Autodesk Inventor part; units mm, degrees
ref_plane "YZ Plane" through (0, 0, 0) normal (1, 0, 0) x (0, 1, 0)
ref_plane "XZ Plane" through (0, 0, 0) normal (0, 1, 0) x (-1, 0, 0)
ref_plane "XY Plane" through (0, 0, 0) normal (0, 0, 1) x (1, 0, 0)
sketch "スケッチ1" plane through (0, 0, 0) normal (0, 0, 1) x (1, 0, 0)
  circle A0 centre (0, 0) radius 1.6
  circle A1 centre (10, 0) radius 1.6
  circle A2 centre (-10, 0) radius 1.6
  circle A3 centre (0, 18) radius 1.6
  circle A4 centre (0, 38) radius 1.6
  circle A5 centre (0, 28) radius 1.6
  line L0 (-17.5, 7.5) -> (-17.5, -7.5)
  line L1 (-17.5, -7.5) -> (17.5, -7.5)
  line L2 (17.5, -7.5) -> (17.5, 7.5)
  line L3 (17.5, 7.5) -> (7.5, 45.5)
  line L4 (7.5, 45.5) -> (-7.5, 45.5)
  line L5 (-7.5, 45.5) -> (-17.5, 7.5)
  dimension "d0" = 3.2
  dimension "d1" = 3.2
  dimension "d2" = 3.2
  dimension "d3" = 10
  dimension "d4" = 10
  dimension "d5" = 3.2
  dimension "d6" = 3.2
  dimension "d7" = 3.2
  dimension "d8" = 18
  dimension "d9" = 10
  dimension "d10" = 10
  dimension "d11" = 7.5
  dimension "d12" = 7.5
  dimension "d13" = 7.5
  dimension "d14" = 7.5
  dimension "d15" = 7.5
  dimension "d16" = 7.5
  dimension "d17" = 7.5
extrude "押し出し1" add sketch "スケッチ1" along normal blind 3
fillet "フィレット1" radius 2 6 edges at (-7.5, 45.5, 1.5) (7.5, 45.5, 1.5) (17.5, 7.5, 1.5) (17.5, -7.5, 1.5) (-17.5, -7.5, 1.5) (-17.5, 7.5, 1.5)
properties part number "オムニ_固定具5" material "アルミニウム 6061"
Geometry check sheet. Reference: the model listing, model coordinates, mm. Round coordinates to 2 decimals unless told otherwise and drop trailing zeros. Loops run counter-clockwise (first coordinate to the right, second up) from the corner with the lowest first, then second, coordinate; pieces in that order, holes last. Notation, with made-up numbers: (-19, 72.5) -> (19, 72.5) arc R33 ccw to (19, 104.5) -> close; hole circle Ø9 at (55, -16.75). An arc over 180 degrees is marked (long way). Use a Markdown table: item, result.
(1) Mould release check, pull along X, two halves, no side actions. Record for faces 1 (the flat face through (12.73, 25.63, 1.48)), 2 (the flat face through (-17.5, 1, 1)), 3 (the cylindrical face through (-11.6, -0.07, 1.48)): released by +X, released by -X, zero draft, split by the parting line, or undercut.
Calculated:
| item | result |
|---|---|
| face 1 | released by +X |
| face 2 | released by -X |
| face 3 | undercut |
(2) Sectioned sample at D-D (y = 33.5). Enter the section's corners in (x, z).
Calculated:
| item | result |
|---|---|
| outline | (-10.66, 0) -> (10.66, 0) -> (10.66, 3) -> (-10.66, 3) -> close |
(3) Sectioned sample at C-C (x = 10). Enter the section's corners in (y, z).
Calculated:
| item | result |
|---|---|
| outline | (-7.5, 0) -> (-1.6, 0) -> (-1.6, 3) -> (-7.5, 3) -> close; (1.6, 0) -> (36, 0) -> (36, 3) -> (1.6, 3) -> close |
(4) Sectioned sample at B-B (z = 1.45). Enter the section's corners in (x, y), then the cut area to 3 significant figures.
Calculated:
| item | result |
|---|---|
| outline | (-17.5, -5.5) arc R2 ccw to (-15.5, -7.5) -> (15.5, -7.5) arc R2 ccw to (17.5, -5.5) -> (17.5, 7.24) arc R2 ccw to (17.43, 7.75) -> (7.89, 44.01) arc R2 ccw to (5.96, 45.5) -> (-5.96, 45.5) arc R2 ccw to (-7.89, 44.01) -> (-17.43, 7.75) arc R2 ccw to (-17.5, 7.24) -> close; hole circle Ø3.2 at (-10, 0); hole circle Ø3.2 at (0, 0); hole circle Ø3.2 at (0, 18); hole circle Ø3.2 at (0, 28); hole circle Ø3.2 at (0, 38); hole circle Ø3.2 at (10, 0) |
| area | 1,420 mm² |
(5) Scan lines: probe 1 along Y at (x, z) = (0, 1.95); probe 2 along X at (y, z) = (39, 2.4); probe 3 along X at (y, z) = (12, 1.95). Record each from-to range of solid material in increasing order.
Calculated:
| item | result |
|---|---|
| probe 1 | -7.5 to -1.6, 1.6 to 16.4, 19.6 to 26.4, 29.6 to 36.4, 39.6 to 45.5 |
| probe 2 | -9.21 to -1.25, 1.25 to 9.21 |
| probe 3 | -16.32 to 16.32 |
(6) Sectioned sample at A-A (x = 0). Enter the section's corners in (y, z), then the cut area to 3 significant figures.
Calculated:
| item | result |
|---|---|
| outline | (-7.5, 0) -> (-1.6, 0) -> (-1.6, 3) -> (-7.5, 3) -> close; (1.6, 0) -> (16.4, 0) -> (16.4, 3) -> (1.6, 3) -> close; (19.6, 0) -> (26.4, 0) -> (26.4, 3) -> (19.6, 3) -> close; (29.6, 0) -> (36.4, 0) -> (36.4, 3) -> (29.6, 3) -> close; (39.6, 0) -> (45.5, 0) -> (45.5, 3) -> (39.6, 3) -> close |
| area | 121 mm² |
(7) Go/stop test with flat-tipped pins: P1, Ø1.9, axis at x = 0, y = 18, coming from the +Z side; P2, Ø1, axis at y = 28.5, z = 2, coming from the -X side. Record where each tip stops, or that it passes through.
Calculated:
| item | result |
|---|---|
| P1 | through |
| P2 | x = -12.11 |
